Could you check a few things on this drawing? It's one solid part, dimensions in mm from its lowest x, y, z. A direction names the side the tool comes from. Round coordinates to 2 decimals unless told otherwise and drop trailing zeros. Write each loop counter-clockwise with the first axis right and the second up, starting at its lowest first coordinate (ties: lowest second). Pieces come first, ordered by that corner, then holes. Notation, with made-up numbers: (-37, -23) - (18, -23) arc R28 ccw to (18, 5) - close; hole circle Ø3 at (0, -8). An arc over 180 degrees is marked (long way). Write item = value, one per line. Start each with the question number.
Item 1: If we section it at B-B (y = 11): Please give me the cut outline in (x, z), and give its area (3 significant figures).
Item 2: If we section it at C-C (z = 1): Please give me the cut outline in (x, y), and give its area (3 significant figures).
Item 3: Which directions (+Z, -Z, +X, -X, +Y, -Y) give clear straight access to the entire face, cutting with the end or side of a thin tool? Please do the marked faces 1 and 2.
Item 4: If we section it at D-D (x = 4.75): Please give me the cut outline in (y, z), and give its area (3 significant figures).
Item 5: For P1, Ø1.5, axis at x = 7.5, y = 11, coming from the -Z side; P2, Ø4, axis at x = 2.5, y = 11, coming from the +Z side, each with a flat end and sliding along its axis, tell me the tip position at first contact or that it passes through.
Item 6: If I drill on line 1 along X through (y, z) = (11, 3.5); line 2 along Y through (x, z) = (4.25, 10); line 3 along Y through (x, z) = (7.5, 4.5), over which ranges is the centre line in solid material (lowest first)? Write a range as [from, to].
Item 7: If we section it at A-A (x = 2.5): Please give me the cut outline in (y, z), and give its area (3 significant figures).
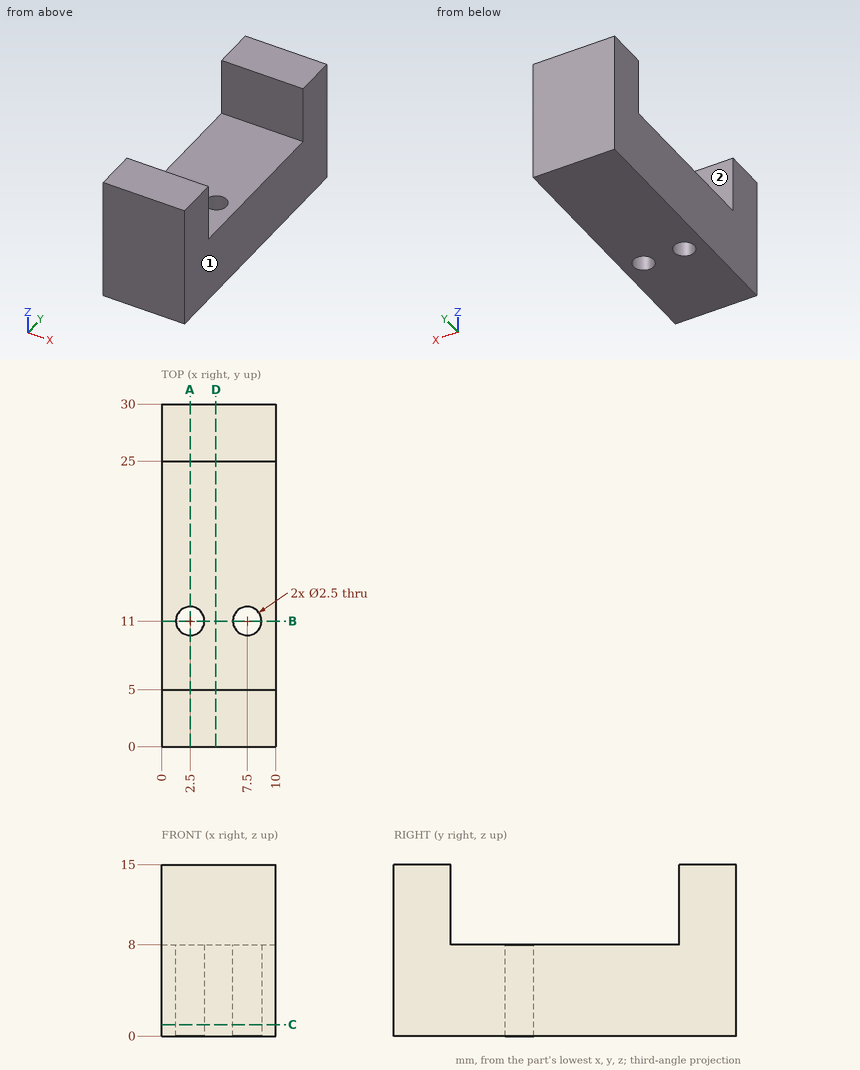
Reply:
q1.outline = (0, 0) - (1.25, 0) - (1.25, 8) - (0, 8) - close; (3.75, 0) - (6.25, 0) - (6.25, 8) - (3.75, 8) - close; (8.75, 0) - (10, 0) - (10, 8) - (8.75, 8) - close
q1.area = 40.0 mm2
q2.outline = (0, 0) - (10, 0) - (10, 30) - (0, 30) - close; hole circle Ø2.5 at (2.5, 11); hole circle Ø2.5 at (7.5, 11)
q2.area = 290 mm2
q3.face_1 = +Z, -Z, +X, +Y, -Y
q3.face_2 = +Z, +X, -X
q4.outline = (0, 0) - (30, 0) - (30, 15) - (25, 15) - (25, 8) - (5, 8) - (5, 15) - (0, 15) - close
q4.area = 310 mm2
q5.P1 = through
q5.P2 = 8
q6.line_1 = [0, 1.25], [3.75, 6.25], [8.75, 10]
q6.line_2 = [0, 5], [25, 30]
q6.line_3 = [0, 9.75], [12.25, 30]
q7.outline = (0, 0) - (9.75, 0) - (9.75, 8) - (5, 8) - (5, 15) - (0, 15) - close; (12.25, 0) - (30, 0) - (30, 15) - (25, 15) - (25, 8) - (12.25, 8) - close
q7.area = 290 mm2
